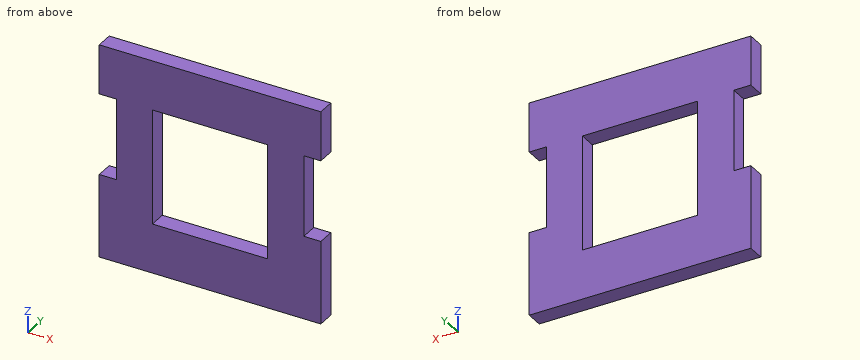
from build123d import *

# Parameters (mm, degrees)
SKETCH1_W           = 41.35
SKETCH1_H           = 40
SKETCH1_W_2         = 21.5
SKETCH1_H_2         = 21.5
BOSS_EXTRUDE1_DEPTH = 3.175
SKETCH2_W           = 3.175
SKETCH2_H           = 15.188
CUT_EXTRUDE1_DEPTH  = 4.175


with BuildPart() as part:
    # Sketch1 → Boss-Extrude1 (new body)
    with BuildSketch(Plane(origin=(0, 0, 0), x_dir=(1, 0, 0), z_dir=(0, 1, 0))):
        with Locations((20.675, 20)):
            Rectangle(SKETCH1_W, SKETCH1_H)
        with Locations((20.675, 20)):
            Rectangle(SKETCH1_W_2, SKETCH1_H_2, mode=Mode.SUBTRACT)
    extrude(amount=BOSS_EXTRUDE1_DEPTH)

    # Sketch2 → Cut-Extrude1 (cut, through all)
    with BuildSketch(Plane(origin=(0, 3.175, 0), x_dir=(1, 0, 0), z_dir=(0, 1, 0))):
        with Locations((39.7625, 16.844)):
            Rectangle(SKETCH2_W, SKETCH2_H)
        with Locations((1.5875, 16.844)):
            Rectangle(SKETCH2_W, SKETCH2_H)
    extrude(amount=-CUT_EXTRUDE1_DEPTH, mode=Mode.SUBTRACT)


solid = part.part
Can you work these out from the model? Positions are in its coordinate system, mm. Coordinates: 2 decimals unless noted, no trailing zeros. Loops run counter-clockwise (first coordinate to the right, second up) from the corner with the lowest first, then second, coordinate; pieces in that order, holes last. Notation, with made-up numbers: M 13,-36.5 L 49,-36.5 A17 ccw 49,-28.5 Z; hole C -6,-9.5 d3. An arc over 180 degrees is marked long. Return JSON: item names as keys, results as strings. Group by question number.
Item 1: Imagine slicing it at B-B (y = 2.65). Please give me the cut outline in (x, z) (3 decimals).
Item 2: If I drill on L1, parallel to Z at x = 40.5, y = 2.7; L2, parallel to X at y = 2.6, z = -21 (3 decimals); L3, parallel to X at y = 0.25, z = -27.5 (3 decimals), over which ranges is the centre line in solid material (lowest first)? Write a range as from..to.
Item 3: I'm going to push flat-ended pins straight in: pin 1 Ø1.6 at (y, z) = (2, -17.5) entering from +X (3 decimals); pin 2 Ø1 at (y, z) = (2.5, -23) entering from -X (3 decimals). Where does each tip first touch, or does it pass through?
Item 4: Imagine slicing it at C-C (x = 20). Please give me the cut outline in (y, z) (3 decimals), and give its area (3 significant figures).
Item 5: Imagine slicing it at A-A (z = -13.5). Please give me the cut outline in (x, y) (3 decimals).
Verdict:
{
 "1": {"outline": "M 0,-40 L 41.35,-40 L 41.35,-24.438 L 38.175,-24.438 L 38.175,-9.25 L 41.35,-9.25 L 41.35,0 L 0,0 L 0,-9.25 L 3.175,-9.25 L 3.175,-24.438 L 0,-24.438 Z; hole M 9.925,-30.75 L 31.425,-30.75 L 31.425,-9.25 L 9.925,-9.25 Z"},
 "2": {"L1": "z = -40..-24.44, -9.25..0", "L2": "x = 3.175..9.925, 31.425..38.175", "L3": "x = 0..9.925, 31.425..41.35"},
 "3": {"pin 1": "stops at x = 38.175", "pin 2": "stops at x = 3.175"},
 "4": {"outline": "M 0,-40 L 3.175,-40 L 3.175,-30.75 L 0,-30.75 Z; M 0,-9.25 L 3.175,-9.25 L 3.175,0 L 0,0 Z", "area": "58.7 mm^2"},
 "5": {"outline": "M 3.175,0 L 9.925,0 L 9.925,3.175 L 3.175,3.175 Z; M 31.425,0 L 38.175,0 L 38.175,3.175 L 31.425,3.175 Z"}
}
